Autodesk Inventor part; units mm, degrees
ref_plane "YZ Plane" through (0, 0, 0) normal (1, 0, 0) x (0, 1, 0)
ref_plane "XZ Plane" through (0, 0, 0) normal (0, 1, 0) x (-1, 0, 0)
ref_plane "XY Plane" through (0, 0, 0) normal (0, 0, 1) x (1, 0, 0)
sketch "Sketch1" plane through (0, 0, 0) normal (0, 0, 1) x (1, 0, 0)
  line L0 (0, 33.6) -> (0, -33.6)
  line L1 (-14, 0) -> (14, 0)
  line L2 (-10, 24) -> (10, 24)
  line L3 (10, 24) -> (10, -24)
  line L4 (10, -24) -> (-10, -24)
  line L5 (-10, -24) -> (-10, 24)
  point P0 (0, 0)
  dimension "d0" = 20
  dimension "d1" = 48
extrude "Extrusion1" add sketch "Sketch1" along normal blind 25
sketch "Sketch2" plane through (0, 0, 25) normal (0, 0, 1) x (1, 0, 0)
  line L0 (0, 49) -> (0, -49)
  line L1 (3, 35) -> (3, -35)
  line L2 (-3, 35) -> (-3, -35)
  line L3 (-10, -24) -> (10, -24)
  line L4 (10, -24) -> (10, 24)
  line L5 (10, 24) -> (-10, 24)
  line L6 (-10, 24) -> (-10, -24)
  point P0 (0, 0)
  point P1 (3, 24)
  point P2 (3, -24)
  point P3 (-3, -24)
  point P4 (-3, 24)
  dimension "d4" = 3
  dimension "d5" = 3
extrude "Extrusion2" cut sketch "Sketch2" against normal blind 1.5 contours L5 L4 L3 L1 | L2 L3 L6 L5
sketch "Sketch3" plane through (10, -24, 0) normal (1, 0, 0) x (0, 0, -1)
  line L0 (-23.5, 48) -> (-23.5, 0)
  line L1 (0, 0) -> (-23.5, 0)
  line L2 (0, 0) -> (0, 48)
  line L3 (0, 48) -> (-23.5, 48)
  line L4 (0, 0) -> (-23.5, 0)
  line L5 (-11.75, 0) -> (-11.75, 48)
  line L6 (0, 48) -> (-23.5, 48)
  line L7 (0, 24) -> (-23.5, 24)
  line L8 (-23.5, 0) -> (-23.5, 48)
  circle A0 centre (-11.75, 24) radius 7
  line L9 (-14.25, 28) -> (-9.25, 28)
  line L10 (-9.25, 28) -> (-9.25, 33)
  line L11 (-9.25, 33) -> (-14.25, 33)
  line L12 (-14.25, 33) -> (-14.25, 28)
  line L13 (-11.75, 17) -> (-11.75, 31)
  line L14 (-12.25, 0) -> (-12.25, 50)
  line L15 (-11.25, 0) -> (-11.25, 50)
  point P0 (-9.25, 30.5383)
  point P1 (-11.25, 33)
  point P2 (-11.25, 48)
  point P3 (-12.25, 48)
  point P4 (-12.25, 33)
  point P5 (-14.25, 30.5383)
  dimension "d8" = 14
  dimension "d9" = 5
  dimension "d10" = 5
  dimension "d11" = 11
  dimension "d12" = 0.5
  dimension "d13" = 0.5
extrude "Extrusion3" cut sketch "Sketch3" against normal through all contours L3 L5 L11 L14 | A0 L12 L9 L14 L7 | L7 L14 A0 | L3 L15 L11 L5 | L14 A0 L12 L11 | L11 L5 A0 L14 | L14 L9 L5 L7 | L7 L5 A0 L14 | A0 L14 L9 L12 | L11 L15 A0 L5 | A0 L5 L9 L14 | L7 L15 A0 L5 | L5 L9 L15 L7 | L11 L10 A0 L15 | A0 L15 L9 L5 | L15 L9 L10 A0 L7 | L7 A0 L15 | A0 L10 L9 L15
sketch "Sketch4" plane through (0, 0, 25) normal (0, 0, 1) x (1, 0, 0)
  line L0 (3, -24) -> (3, 24)
  line L1 (3, 24) -> (-3, 24)
  line L2 (-3, 24) -> (-3, -24)
  line L3 (-3, -24) -> (3, -24)
  line L4 (0, 35) -> (0, -35)
  circle A0 centre (0, 16) radius 3
  circle A1 centre (0, -16) radius 3
  line L5 (-10, 6.5383) -> (-10, 9)
  line L6 (10, 6.5383) -> (-10, 6.5383)
  line L7 (10, 9) -> (10, 6.5383)
  line L8 (10, 9) -> (-10, 9)
  line L9 (10, 6.5383) -> (-10, 6.5383)
  line L10 (10, -7) -> (-10, -7)
  line L11 (-10, 6.5383) -> (-10, 6.5383)
  line L12 (10, 6.5383) -> (-10, 6.5383)
  line L13 (10, 6.5383) -> (10, 6.5383)
  line L14 (10, 6.5383) -> (-10, 6.5383)
  line L15 (10, 6.5383) -> (10, -7)
  line L16 (-10, -7) -> (-10, 6.5383)
  point P0 (0, 0)
  dimension "d16" = 6
  dimension "d17" = 6
  dimension "d18" = 8
  dimension "d19" = 8
extrude "Extrusion4" cut sketch "Sketch4" against normal through all contours A1 L4 | L4 A1 | A0 L4 | L4 A0
properties part number "motor shaft clamp"
Check sheet for the modelled part. Datum: model origin and axes. Units: mm. A direction names the side the tool comes from. Give positions to 0.01 mm unless a question says otherwise; leave off trailing zeros. Write each loop counter-clockwise with the first axis right and the second up, starting at its lowest first coordinate (ties: lowest second). Pieces come first, ordered by that corner, then holes.
Item 1: Draft check along Y on faces 6 (the face through (0, 8, 14.25)), 7 (the face through (0, -21, 25)), 8 (the face through (0, 24, 6)). Enter one of: released by +Y, released by -Y, zero draft, split by the parting line, or undercut.
Item 2: Cross-section at C-C (x = 0). Enter the section's corners in (y, z).
Item 3: Scan lines: L1, parallel to Y at x = 0, z = 2.5; L2, parallel to X at y = 16, z = 20; L3, parallel to Z at x = -5, y = 15. Record each from-to range of solid material in increasing order.
Item 4: Access from +Z, -Z, +X, -X, +Y, -Y to the whole of each face (thin tool, end or side, straight path). Record for faces 1 (the face through (0, 21, 25)), 2 (the face through (0, 9, 10)), 3 (the face through (2.4, 18.1, 12.25)), 4 (the face through (3, 0, 24)), 5 (the face through (-3, 0, 24)).
Item 5: Cross-section at B-B (y = 8). Enter the section's corners in (x, z), and give its area (3 significant figures).
Item 6: Cross-section at A-A (z = 15.5). Enter the section's corners in (x, y), and give its area (3 significant figures).
Item 7: Gauge pin test, flat ends, axial feed: pin 1 (1.2 mm diameter, centred on y = 19.5, z = 24.5, fed in from +X); pin 2 (5 mm diameter, centred on x = 0, y = -16, fed in from -Z); pin 3 (2 mm diameter, centred on x = 5.5, y = 2.5, fed in from +Z). Record the tip position at first contact, or that the pin passes through.
Item 8: Cross-section at D-D (x = 4.75). Enter the section's corners in (y, z).
Report:
1. face 6: undercut
1. face 7: zero draft
1. face 8: released by +Y
2. outline: (-24, 0) - (-19, 0) - (-19, 25) - (-24, 25) - close; (-13, 0) - (13, 0) - (13, 11.25) - (9, 11.25) - (9, 9.25) - (6.54, 9.25) arc R7 cw (long way) to (6.54, 14.25) - (9, 14.25) - (9, 12.25) - (13, 12.25) - (13, 25) - (-13, 25) - close; (19, 0) - (24, 0) - (24, 11.25) - (19, 11.25) - close; (19, 12.25) - (24, 12.25) - (24, 25) - (19, 25) - close
3. L1: y = -24 to -19, -13 to 13, 19 to 24
3. L2: x = -10 to -3, 3 to 10
3. L3: z = 0 to 11.25, 12.25 to 23.5
4. face 1: +Z, +X, -X, +Y, -Y
4. face 2: +X, -X
4. face 3: +X, -X, +Y
4. face 4: +Z, +X, +Y, -Y
4. face 5: +Z, -X, +Y, -Y
5. outline: (-10, 0) - (10, 0) - (10, 9.25) - (-10, 9.25) - close; (-10, 14.25) - (10, 14.25) - (10, 23.5) - (3, 23.5) - (3, 25) - (-3, 25) - (-3, 23.5) - (-10, 23.5) - close
5. area: 379 mm2
6. outline: (-10, -24) - (10, -24) - (10, -5.91) - (-10, -5.91) - close; (-10, 5.91) - (10, 5.91) - (10, 24) - (-10, 24) - close; hole circle Ø6 at (0, -16); hole circle Ø6 at (0, 16)
6. area: 667 mm2
7. pin 1: stops at x = 3
7. pin 2: passes through
7. pin 3: stops at z = 23.5
8. outline: (-24, 0) - (24, 0) - (24, 11.25) - (9, 11.25) - (9, 9.25) - (6.54, 9.25) arc R7 cw (long way) to (6.54, 14.25) - (9, 14.25) - (9, 12.25) - (24, 12.25) - (24, 23.5) - (-24, 23.5) - close
